```python
from build123d import *

# Parameters (mm, degrees)
SKETCH_R             = 4
PAD_DEPTH            = 12
SKETCH001_R          = 15
PAD001_DEPTH         = 45
PAD002_DEPTH         = 4
SKETCH003_R          = 7.5
POCKET_DEPTH         = 57.001
SKETCH004_R          = 4
SKETCH004_W          = 8
SKETCH004_H          = 5
POCKET001_DEPTH      = 25.001
POCKET001_DEPTH_BACK = -25.001


with BuildPart() as part:
    # Sketch → Pad (new body)
    with BuildSketch(Plane.XZ):
        with BuildLine():
            ThreePointArc((-42, 25), (-47.656854, 22.656854), (-50, 17))
            Line((-50, -17), (-50, 17))
            ThreePointArc((-50, -17), (-47.656854, -22.656854), (-42, -25))
            Line((42, -25), (-42, -25))
            ThreePointArc((42, -25), (47.656854, -22.656854), (50, -17))
            Line((50, 17), (50, -17))
            ThreePointArc((50, 17), (47.656854, 22.656854), (42, 25))
            Line((-42, 25), (42, 25))
        make_face()
        with Locations((-42, 17)):
            Circle(SKETCH_R, mode=Mode.SUBTRACT)
        with Locations((-42, -17)):
            Circle(SKETCH_R, mode=Mode.SUBTRACT)
        with Locations((42, 17)):
            Circle(SKETCH_R, mode=Mode.SUBTRACT)
        with Locations((42, -17)):
            Circle(SKETCH_R, mode=Mode.SUBTRACT)
    extrude(amount=PAD_DEPTH)

    # Sketch001 (on Face14 of Pad) → Pad001 (join)
    with BuildSketch(Plane.XZ.offset(12)):
        Circle(SKETCH001_R)
    extrude(amount=PAD001_DEPTH)

    # Sketch002 → Pad002 (join, symmetric)
    with BuildSketch(Plane.XY):
        Polygon((-5.727757, -32), (-14.773027, -32), (-50, -12), (-5.727757, -12), align=None)
    pad002 = extrude(amount=PAD002_DEPTH, both=True)

    # Mirrored: Pad002 across Sketch002 V_Axis
    add(pad002.mirror(Plane(origin=(0, 0, 0), x_dir=(0, 0, 1), z_dir=(1, 0, 0))))

    # Sketch003 (on Face26 of Mirrored) → Pocket (cut, through all)
    with BuildSketch(Plane.XZ.offset(57)):
        Circle(SKETCH003_R)
    extrude(amount=-POCKET_DEPTH, mode=Mode.SUBTRACT)

    # Sketch004 → Pocket001 (cut, two sides)
    with BuildSketch(Plane.XY) as pocket001_sk:
        with Locations((0, -22)):
            Circle(SKETCH004_R)
        with Locations((0, -54.5)):
            Rectangle(SKETCH004_W, SKETCH004_H)
    extrude(amount=-POCKET001_DEPTH, mode=Mode.SUBTRACT)
    extrude(pocket001_sk.sketch, amount=-POCKET001_DEPTH_BACK, mode=Mode.SUBTRACT)


solid = part.part
```
Geometry check sheet. Reference: the model listing, model coordinates, mm. A direction names the side the tool comes from. Give positions to 0.01 mm unless a question says otherwise; leave off trailing zeros. Loops run counter-clockwise (first coordinate to the right, second up) from the corner with the lowest first, then second, coordinate; pieces in that order, holes last. Notation, with made-up numbers: M 38.25,-17 L 71.25,-17 A14 cw 71.25,-8 Z; hole C 81.25,-35 d2. An arc over 180 degrees is marked long. Write item = value, one per line.
(1) Release check for a two-part mould opening along Z. For faces 6 (the face through (47.594, -5.916, -22.719)), 7 (the face through (-44.95, -5.92, -14.3)), 8 (the face through (-1, 0, 11)) record: released by +Z, released by -Z, zero draft, split by the parting line, or undercut.
Answer below:
face_6 = released by -Z
face_7 = undercut
face_8 = zero draft
(2) Gauge pin test, flat ends, axial feed: pin 1 Ø13 at (x, z) = (-42, 17) entering from -Y; pin 2 Ø1.5 at (y, z) = (-20.5, 0.5) entering from +X; pin 3 Ø12 at (y, z) = (-44, -4) entering from -X. Record the tip position at first contact, or that the pin passes through.
Answer below:
pin_1 = -12
pin_2 = 36.35
pin_3 = -15
(3) Sectioned sample at C-C, the plane x = 39.5. Record the cut outline in (y, z), plus the area to 3 significant figures.
Answer below:
outline = M -17.96,-4 L -12,-4 L -12,-13.88 L 0,-13.88 L 0,13.88 L -12,13.88 L -12,4 L -17.96,4 Z; M -12,-25 L 0,-25 L 0,-20.12 L -12,-20.12 Z; M -12,20.12 L 0,20.12 L 0,25 L -12,25 Z
area = 498 mm2
(4) Sectioned sample at A-A, the plane x = 0. Record the cut outline in (y, z).
Answer below:
outline = M -52,-15 L -26,-15 L -26,-7.5 L -52,-7.5 Z; M -52,7.5 L -26,7.5 L -26,15 L -52,15 Z; M -18,-15 L -12,-15 L -12,-25 L 0,-25 L 0,-7.5 L -18,-7.5 Z; M -18,7.5 L 0,7.5 L 0,25 L -12,25 L -12,15 L -18,15 Z
(5) Material ranges on line 1 (Z direction, x = -42, y = -7.5); line 2 (X direction, y = -38.5, z = 4); line 3 (X direction, y = -11.5, z = -16), recorded low to high. Write a range as [from, to].
Answer below:
line_1 = [-25, -21], [-13, 13], [21, 25]
line_2 = [-14.46, -6.34], [6.34, 14.46]
line_3 = [-50, -45.87], [-38.13, 38.13], [45.87, 50]
(6) Sectioned sample at B-B, the plane y = -45.5. Record the cut outline in (x, z), plus the area to 3 significant figures.
Answer below:
outline = C 0,0 d30; hole C 0,0 d15
area = 530 mm2
(7) Tool access check on faces 1 (the face through (13.856, -34.185, -5.745)), 2 (the face through (28, -20, 4)), 3 (the face through (-28, -20, -4)), 4 (the face through (4, -55, -10)), 5 (the face through (-1, -12, -17)). Record the directions out of +Z, -Z, +X, -X, +Y, -Y that give a thin tool (end or side, any length) a straight path to the whole face; none if there is none.
Answer below:
face_1 = -Y
face_2 = +Z, +X, -Y
face_3 = -Z, -X, -Y
face_4 = +Z, -Z, -Y
face_5 = -Z, -Y
(8) Sectioned sample at D-D, the plane z = 0. Record the cut outline in (x, y), plus the area to 3 significant figures.
Answer below:
outline = M -50,-12 L -15,-31.87 L -15,-57 L -7.5,-57 L -7.5,0 L -50,0 Z; M 7.5,-57 L 15,-57 L 15,-31.87 L 50,-12 L 50,0 L 7.5,0 Z
area = 2,390 mm2
